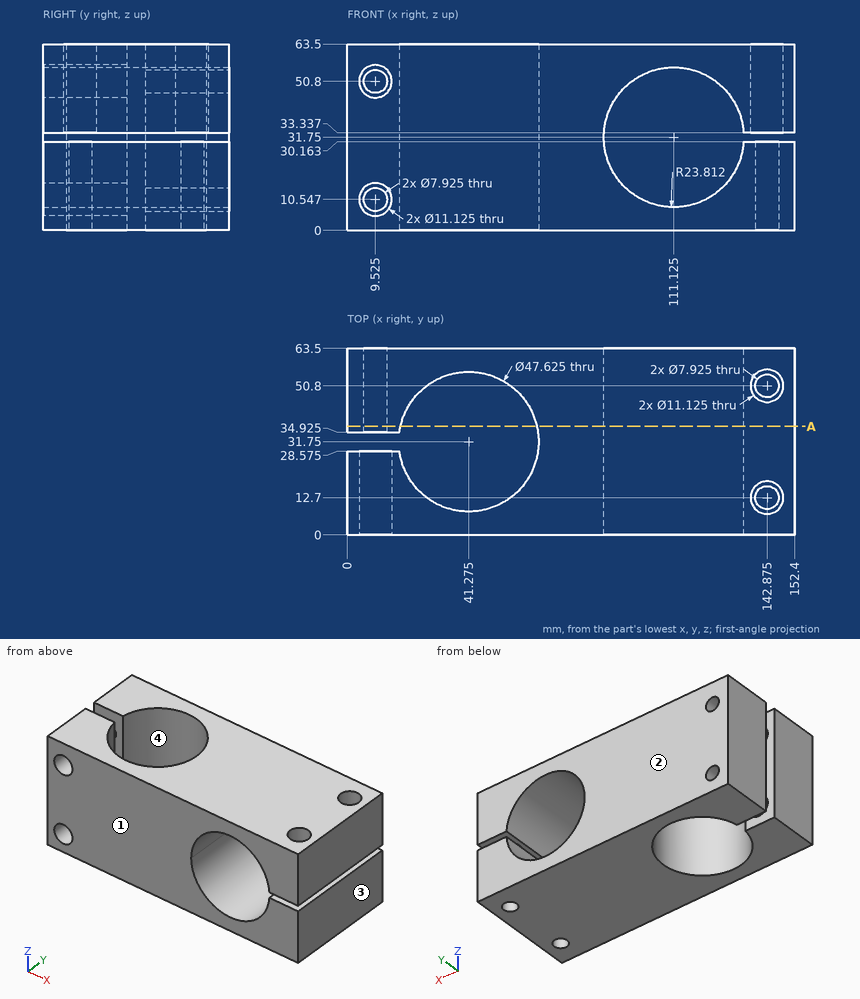
Input: dimensioned drawing with shaded views. Units: mm. Origin: part minimum x, y, z. Coordinates: 2 decimals unless noted, no trailing zeros. Return JSON: item names as keys, results as strings. Group by question number.
1. Cut plane A-A (y = 37). Count the separate pieces of the cut face and the enclosed holes in it, plus the area to 3 significant figures.
2. Pull-direction query (Y, two-part tool) for the marked faces 1, 2, 3 and 4; classes: pulls with the +Y half, pulls with the -Y half, needs draft (parallel to the pull), parting line crosses it, or undercut.
3. Material intervals for line 1 along X through (y, z) = (13, 3.5) (1 decimal); line 2 along Y through (x, z) = (144, 51); line 3 along X through (y, z) = (13.5, 41) (1 decimal), sorted ascending. Write a range as [from, to].
4. Pin query (flat end, axial travel): pin 1 (5 mm diameter, centred on x = 9.53, z = 10.55, fed in from -Y). Return the tip coordinate at first contact, or that it passes through.
Resolved:
{
 "1": {"separate pieces": "2", "enclosed holes": "2", "area": "4,790 mm²"},
 "2": {"face 1": "pulls with the -Y half", "face 2": "pulls with the +Y half", "face 3": "needs draft", "face 4": "undercut"},
 "3": {"line 1": "x = [0, 26.6], [56, 138.9], [146.8, 152.4]", "line 2": "y = [0, 7.25], [18.15, 45.35], [56.25, 63.5]", "line 3": "x = [0, 26], [56.6, 89.2], [133.1, 137.4], [148.4, 152.4]"},
 "4": {"pin 1": "passes through"}
}
